Autodesk Fusion 360 part; units mm, degrees
sketch "Sketch1" plane through (0, 0, 0) normal (0, 0, 1) x (1, 0, 0)
  line L0 (0, 0) -> (150, 0)
  line L1 (150, 0) -> (150, 140)
  line L2 (150, 140) -> (0, 140)
  line L3 (0, 140) -> (0, 0)
  dimension "d1" = 150
  dimension "d2" = 140
extrude "Extrude1" add sketch "Sketch1" along normal blind 5
sketch "Sketch2" plane through (0, 0, 5) normal (0, 0, 1) x (-1, 0, 0)
  line L0 (0, -140) -> (0, 0)
  line L1 (0, 0) -> (-150, 0)
  line L2 (-150, 0) -> (-150, -140)
  line L3 (-150, -140) -> (0, -140)
  line L4 (0, -140) -> (-150, -140)
  line L5 (-150, -140) -> (-150, -135)
  line L6 (-150, -135) -> (0, -135)
  line L7 (0, -135) -> (0, -140)
  line L8 (0, 0) -> (-150, 0)
  line L9 (-150, 0) -> (-150, -5)
  line L10 (-150, -5) -> (0, -5)
  line L11 (0, -5) -> (0, 0)
  line L12 (-75, -140) -> (-77, -140)
  line L13 (-77, -140) -> (-77, -135)
  line L14 (-77, -135) -> (-75, -135)
  line L15 (-75, -135) -> (-75, -140)
  line L16 (-75, 0) -> (-77, 0)
  line L17 (-77, 0) -> (-77, -5)
  line L18 (-77, -5) -> (-75, -5)
  line L19 (-75, -5) -> (-75, 0)
  dimension "d5" = 2
  dimension "d6" = 5
  dimension "d7" = 2
  dimension "d8" = 5
extrude "Extrude2" add sketch "Sketch2" along normal blind 20 contours L0 L3 L4 L6 L7 L15 | L0 L1 L8 L10 L11 L19 | L2 L3 L4 L5 L6 L13 | L1 L2 L8 L9 L10 L17
sketch "Sketch3" plane through (0, 0, 5) normal (0, 0, 1) x (-1, 0, 0)
  line L0 (-77, -5) -> (-150, -5)
  line L1 (-150, -5) -> (-150, -135)
  line L2 (-150, -135) -> (-77, -135)
  line L3 (-77, -135) -> (-77, -140)
  line L4 (-77, -140) -> (-75, -140)
  line L5 (-75, -140) -> (-75, -135)
  line L6 (-75, -135) -> (0, -135)
  line L7 (0, -135) -> (0, -5)
  line L8 (0, -5) -> (-75, -5)
  line L9 (-75, -5) -> (-75, 0)
  line L10 (-75, 0) -> (-77, 0)
  line L11 (-77, 0) -> (-77, -5)
  line L12 (-75, -140) -> (-77, -140)
  line L13 (-77, -140) -> (-77, 0)
  line L14 (-77, 0) -> (-75, 0)
  line L15 (-75, 0) -> (-75, -140)
  dimension "d11" = 2
  dimension "d12" = 140
extrude "Extrude3" cut sketch "Sketch3" against normal blind 2 contours L3 L4 L5 L9 L10 L11 L12 L13 L14 L15
chamfer "Chamfer1" distance 5 angle 45 4 edges at (75, 2.5, 25) (77, 2.5, 25) (75, 137.5, 25) (77, 137.5, 25)
chamfer "Chamfer2" distance 25 angle 45 4 edges at (150, 2.5, 25) (150, 137.5, 25) (0, 2.5, 25) (0, 137.5, 25)
Part model, mm, in its own coordinate system. A direction names the side the tool comes from. Round coordinates to 2 decimals unless told otherwise and drop trailing zeros. Order: outer loops, then holes, each group sorted by start corner. A loop starts at its lowest first (then second) coordinate and runs counter-clockwise, first axis right, second up. Notation, with made-up numbers: M -20,81 L -3,81 A21 cw -3,116 Z; hole C 6,67 d6. An arc over 180 degrees is marked long. Answer in a Markdown table with one row per item. Add a question column.
Q1. Wall check: L1, parallel to Y at x = 63, z = 7; L2, parallel to Z at x = 42, y = 46.5; L3, parallel to X at y = 44, z = 4.75 (3 decimals). Give the ranges that are in metal, low to high. Write a range as from..to.
Q2. Cut at B-B on y = 98. Give the cut face in (x, z) (3 decimals), and give its area (3 significant figures).
Q3. 3-axis set-ups, long thin cutter, end or side, ignore diameter. For faces 1 (the face through (73, 2, 22)), 2 (the face through (104, 135, 15)), 3 (the face through (76, 140, 1)): which of +Z, -Z, +X, -X, +Y, -Y reach the whole face in a straight line?
Q4. Cut at A-A on z = 17.25. Give the cut face in (x, y) (3 decimals), and give its area (3 significant figures).
Q5. Cut at C-C on x = 95.5. Give the cut face in (y, z), and give its area (3 significant figures).
Q6. Mould opens along X. For faces 4 (the face through (146.702, 70.327, 3.303)), 5 (the face through (40, 135, 15)), 6 (the face through (75, 69.7, 4.5)) say: +X half, -X half, draft (parallel to the pull), parting line (faces both ways), or undercut.
Q7. Cut at D-D on z = 7.75. Give the cut face in (x, y) (3 decimals).
Q8. Pin check, flat tips, straight feed: pin 1 (8 mm diameter, centred on x = 30, y = 119.5, fed in from +Z); pin 2 (13.5 mm diameter, centred on y = 86, z = 15.5, fed in from +X); pin 3 (0.6 mm diameter, centred on x = 76.5, y = 50.5, fed in from +Z). Stop position of each tip, or through.
Established:
| question | item | result |
|---|---|---|
| 1 | L1 | y = 0..5, 135..140 |
| 1 | L2 | z = 0..5 |
| 1 | L3 | x = 4.745..75, 77..145.255 |
| 2 | outline | M 0,0 L 150,0 L 150,0.005 L 145.005,5 L 77,5 L 77,3 L 75,3 L 75,5 L 4.995,5 L 0,0.005 Z |
| 2 | area | 721 mm2 |
| 3 | face 1 | +Z, +Y, -Y |
| 3 | face 2 | +Z, +X, -X |
| 3 | face 3 | +Z, -Z, +X, -X, +Y |
| 4 | outline | M 17.245,0 L 75,0 L 75,5 L 17.245,5 Z; M 17.245,135 L 75,135 L 75,140 L 17.245,140 Z; M 77,0 L 132.755,0 L 132.755,5 L 77,5 Z; M 77,135 L 132.755,135 L 132.755,140 L 77,140 Z |
| 4 | area | 1,140 mm2 |
| 5 | outline | M 0,0 L 140,0 L 140,25 L 135,25 L 135,5 L 5,5 L 5,25 L 0,25 Z |
| 5 | area | 900 mm2 |
| 6 | face 4 | +X half |
| 6 | face 5 | draft |
| 6 | face 6 | undercut |
| 7 | outline | M 7.745,0 L 75,0 L 75,5 L 7.745,5 Z; M 7.745,135 L 75,135 L 75,140 L 7.745,140 Z; M 77,0 L 142.255,0 L 142.255,5 L 77,5 Z; M 77,135 L 142.255,135 L 142.255,140 L 77,140 Z |
| 8 | pin 1 | stops at z = 5 |
| 8 | pin 2 | passes through |
| 8 | pin 3 | stops at z = 3 |
